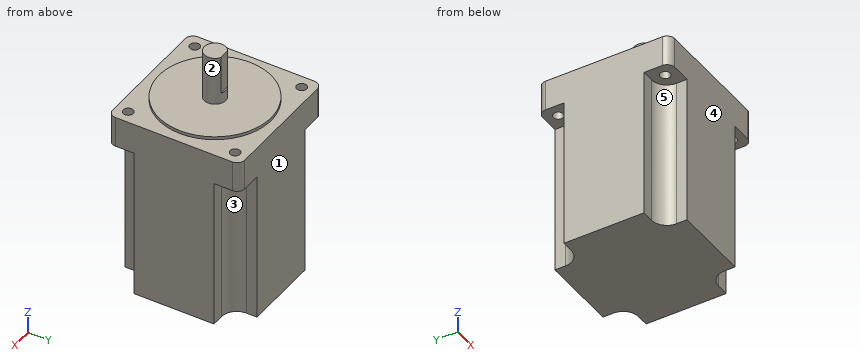
from build123d import *

# Parameters (mm, degrees)
SKETCH_1_W          = 86
SKETCH_1_H          = 86
EXTRUDE_1_DEPTH     = 118
FILLET_1_R          = 5
SKETCH_2_R          = 36.5
EXTRUDE_2_DEPTH     = 2
SKETCH_3_R          = 7
EXTRUDE_3_DEPTH     = 32
SKETCH_4_W          = 6.847911944
SKETCH_4_H          = 3.276194793
CUT_EXTRUDE_1_DEPTH = 25
SKETCH_5_R          = 3.25
CUT_EXTRUDE_2_DEPTH = 119
CUT_EXTRUDE_3_DEPTH = 98


with BuildPart() as part:
    # 草图1 → 凸台-拉伸1 (new body)
    with BuildSketch(Plane.XY):
        with Locations((43, 43)):
            Rectangle(SKETCH_1_W, SKETCH_1_H)
    extrude(amount=EXTRUDE_1_DEPTH)

    # 圆角1
    fillet_1_edges = [part.edges().sort_by_distance(p)[0] for p in [
        (0, 86, 59),
        (86, 86, 59),
        (86, 0, 59),
        (0, 0, 59),
    ]]
    fillet(fillet_1_edges, radius=FILLET_1_R)

    # 草图2 → 凸台-拉伸2 (add)
    with BuildSketch(Plane.XY.offset(118)):
        with Locations((43, 43)):
            Circle(SKETCH_2_R)
    extrude(amount=EXTRUDE_2_DEPTH)

    # 草图3 → 凸台-拉伸3 (add)
    with BuildSketch(Plane.XY.offset(120)):
        with Locations((43, 43)):
            Circle(SKETCH_3_R)
    extrude(amount=EXTRUDE_3_DEPTH)

    # 草图4 → 切除-拉伸1 (cut)
    with BuildSketch(Plane.XY.offset(152)):
        with Locations((43, 50.638097397)):
            Rectangle(SKETCH_4_W, SKETCH_4_H)
    extrude(amount=-CUT_EXTRUDE_1_DEPTH, mode=Mode.SUBTRACT)

    # 草图5 → 切除-拉伸2 (cut, through all)
    with BuildSketch(Plane.XY.offset(118)):
        with Locations((8.2, 77.8)):
            Circle(SKETCH_5_R)
        with Locations((77.8, 77.8)):
            Circle(SKETCH_5_R)
        with Locations((77.8, 8.2)):
            Circle(SKETCH_5_R)
        with Locations((8.2, 8.2)):
            Circle(SKETCH_5_R)
    extrude(amount=-CUT_EXTRUDE_2_DEPTH, mode=Mode.SUBTRACT)

    # 草图6 → 切除-拉伸3 (cut)
    with BuildSketch(Plane(origin=(0, 0, 0), x_dir=(-1, 0, 0), z_dir=(0, 0, -1))):
        with BuildLine():
            Line((-68.156525259, 86), (-93.025218422, 86))
            Line((-93.025218422, 86), (-93.025218422, 69.077587969))
            Line((-93.025218422, 69.077587969), (-78.156525259, 69.077587969))
            ThreePointArc((-78.156525259, 69.077587969), (-71.085457448, 72.006520157), (-68.156525259, 79.077587969))
            Line((-68.156525259, 79.077587969), (-68.156525259, 86))
        make_face()
        with BuildLine():
            Line((-17.843474741, 86), (-17.843474741, 79.077587969))
            ThreePointArc((-17.843474741, 79.077587969), (-14.914542552, 72.006520157), (-7.843474741, 69.077587969))
            Line((-7.843474741, 69.077587969), (7.025218422, 69.077587969))
            Line((7.025218422, 69.077587969), (7.025218422, 86))
            Line((7.025218422, 86), (-17.843474741, 86))
        make_face()
        with BuildLine():
            Line((-7.843474741, 16.922412031), (7.025218422, 16.922412031))
            Line((7.025218422, 16.922412031), (7.025218422, 0))
            Line((7.025218422, 0), (-17.843474741, 0))
            Line((-17.843474741, 0), (-17.843474741, 6.922412031))
            ThreePointArc((-17.843474741, 6.922412031), (-14.914542552, 13.993479843), (-7.843474741, 16.922412031))
        make_face()
        with BuildLine():
            Line((-68.156525259, 0), (-68.156525259, 6.922412031))
            ThreePointArc((-68.156525259, 6.922412031), (-71.085457448, 13.993479843), (-78.156525259, 16.922412031))
            Line((-78.156525259, 16.922412031), (-93.025218422, 16.922412031))
            Line((-93.025218422, 16.922412031), (-93.025218422, 0))
            Line((-93.025218422, 0), (-68.156525259, 0))
        make_face()
    extrude(amount=-CUT_EXTRUDE_3_DEPTH, mode=Mode.SUBTRACT)


solid = part.part
Model file for the job. Use its own axes, mm. Face numbers are marked on the shaded views. A direction names the side the tool comes from. Give positions to 0.01 mm unless a question says otherwise; leave off trailing zeros. Loops run counter-clockwise (first coordinate to the right, second up) from the corner with the lowest first, then second, coordinate; pieces in that order, holes last.
1) Saw through at A-A (z = 85.5). Write the cut outline in (x, y), plus the area to 3 significant figures.
2) Saw through at C-C (z = 112.5). Write the cut outline in (x, y).
3) Tool access for the marked faces 1, 2, 3, 4 and 5: list every direction of +Z, -Z, +X, -X, +Y, -Y with a clear straight run to the whole face (end or side of a thin tool).
4) Saw through at D-D (y = 43). Write the cut outline in (x, z), plus the area to 3 significant figures.
5) Flat gauge pins, fed straight in: pin 1 Ø6 at (x, y) = (8.2, 77.8) entering from +Z (1 decimal); pin 2 Ø2.5 at (x, z) = (83, 30) entering from -Y; pin 3 Ø7.5 at (y, z) = (3.5, 30) entering from -X; pin 4 Ø5.5 at (y, z) = (83.5, 25) entering from +X. Where does each tip first touch, or does it go through?
6) Saw through at B-B (x = 43). Write the cut outline in (y, z), plus the area to 3 significant figures.
7) Wall check: line 1 (Y direction, x = 77.8, z = 112); line 2 (X direction, y = 8, z = 106); line 3 (Z direction, x = 56.5, y = 24.5). Give the ranges that are in metal, low to high.
Answer block:
1. outline: (0, 16.92) - (7.84, 16.92) arc R10 cw to (17.84, 6.92) - (17.84, 0) - (68.16, 0) - (68.16, 6.92) arc R10 cw to (78.16, 16.92) - (86, 16.92) - (86, 69.08) - (78.16, 69.08) arc R10 cw to (68.16, 79.08) - (68.16, 86) - (17.84, 86) - (17.84, 79.08) arc R10 cw to (7.84, 69.08) - (0, 69.08) - close
1. area: 6,270 mm2
2. outline: (0, 5) arc R5 ccw to (5, 0) - (81, 0) arc R5 ccw to (86, 5) - (86, 81) arc R5 ccw to (81, 86) - (5, 86) arc R5 ccw to (0, 81) - close; hole circle Ø6.5 at (8.2, 8.2); hole circle Ø6.5 at (8.2, 77.8); hole circle Ø6.5 at (77.8, 8.2); hole circle Ø6.5 at (77.8, 77.8)
3. face 1: +Z, -Z, +X, -X, +Y
3. face 2: +Z
3. face 3: -Z, +X, +Y
3. face 4: +Z, -Z, +X, -X, -Y
3. face 5: -Z, -X, -Y
4. outline: (0, 0) - (86, 0) - (86, 118) - (79.5, 118) - (79.5, 120) - (50, 120) - (50, 152) - (36, 152) - (36, 120) - (6.5, 120) - (6.5, 118) - (0, 118) - close
4. area: 10,700 mm2
5. pin 1: passes through
5. pin 2: stops at y = 16.92
5. pin 3: stops at x = 17.84
5. pin 4: stops at x = 68.16
6. outline: (0, 0) - (86, 0) - (86, 118) - (79.5, 118) - (79.5, 120) - (50, 120) - (50, 127) - (49, 127) - (49, 152) - (36, 152) - (36, 120) - (6.5, 120) - (6.5, 118) - (0, 118) - close
6. area: 10,700 mm2
7. line 1: y = 0 to 4.95, 11.45 to 74.55, 81.05 to 86
7. line 2: x = 0 to 4.96, 11.44 to 74.56, 81.04 to 86
7. line 3: z = 0 to 120
